Source: CAD feature listing. Evaluate the final solid. Frame: model axes, mm. A direction names the side the tool comes from. Give positions to 0.01 mm unless a question says otherwise; leave off trailing zeros. Order: outer loops, then holes, each group sorted by start corner. A loop starts at its lowest first (then second) coordinate and runs counter-clockwise, first axis right, second up. Notation, with made-up numbers: M -15,72 L 34,72 A21 ccw 34,101 Z; hole C 18,50 d8. An arc over 180 degrees is marked long. Answer in a Markdown table with one row per item. Add a question column.
(1) Section query A-A, the plane y = 31.5. Return loops of the section in (x, z).
(2) Section query C-C, the plane x = -31.5. Return loops of the section in (y, z), plus the area to 3 significant figures.
(3) Pin query (flat end, axial travel): P1, Ø2, axis at y = 27.5, z = 38.5, coming from the +X side; P2, Ø7, axis at x = -29.34, y = 31.5, coming from the -Z side; P3, Ø1, axis at y = 26.5, z = 8, coming from the -X side; P4, Ø4, axis at x = -45.74, z = 50.2, coming from the +Y side. Return the tip coordinate at first contact, or that it passes through.
(4) Mould query, pull axis Y, two halves, no side actions, for faces 1 (the face through (-47.31, 24.36, 51.75)), 2 (the face through (-28.72, 36.21, -11.17)), 3 (the face through (-29, 37.6, 11)), 4 (the face through (-31.3, 27.73, -11.33)). Classes: pulls with the +Y half, pulls with the -Y half, needs draft (parallel to the pull), parting line crosses it, or undercut.
(5) Section query B-B, the plane z = -3. Return loops of the section in (x, y), plus the area to 3 significant figures.
(6) Set-up query: faces 5 (the face through (-25, 29, -5.5)), 6 (the face through (-29, 25.1, 5)), 7 (the face through (-22.041, 31, 11)). Return all of +Z, -Z, +X, -X, +Y, -Y with unobstructed straight access to the full face (end or side cutting, diameter ignored); none if empty.
(7) Section query D-D, the plane y = 28. Return loops of the section in (x, z), plus the area to 3 significant figures.
(8) Material intervals for line 1 along Y through (x, z) = (-22, 19); line 2 along X through (y, z) = (36.75, 9.5); line 3 along Z through (x, y) = (-33, 24.5), sorted ascending.
from build123d import *

# Parameters (mm, degrees)
EXTRUDE_1_DEPTH      = 3.5
EXTRUDE_1_DEPTH_BACK = 5.5
SKETCH_1_R           = 6
SKETCH_2_R           = 4.75
EXTRUDE_2_DEPTH      = 11.5
SKETCH_3_R           = 4.25
CUT_EXTRUDE_1_DEPTH  = 11.5
SKETCH_4_W           = 14.6
SKETCH_4_H           = 12.5
EXTRUDE_3_DEPTH      = 14.2
SKETCH_5_R           = 1.25
EXTRUDE_4_DEPTH      = 1.5


with BuildPart() as part:
    # 草圖1 → 填料-伸長1 (new, two sides: drawn at the far end of the back side and taken through both)
    with BuildSketch(Plane.XY.offset(-EXTRUDE_1_DEPTH_BACK)):
        with Locations((-29.340909091, 31.5)):
            Circle(SKETCH_1_R)
    extrude(amount=EXTRUDE_1_DEPTH + EXTRUDE_1_DEPTH_BACK)

    # 草圖2 → 填料-伸長2 (add)
    with BuildSketch(Plane(origin=(0, 0, -5.5), x_dir=(-1, 0, 0), z_dir=(0, 0, -1))):
        with Locations((29.340909091, 31.5)):
            Circle(SKETCH_2_R)
    extrude(amount=EXTRUDE_2_DEPTH)

    # 草圖3 → 除料-伸長1 (cut)
    with BuildSketch(Plane(origin=(0, 0, -17), x_dir=(-1, 0, 0), z_dir=(0, 0, -1))):
        with Locations((29.340909091, 31.5)):
            Circle(SKETCH_3_R)
    extrude(amount=-CUT_EXTRUDE_1_DEPTH, mode=Mode.SUBTRACT)

    # 草圖4 → 填料-伸長3 (add)
    with BuildSketch(Plane.XY.offset(3.5)):
        with Locations((-29.340909091, 31.35)):
            Rectangle(SKETCH_4_W, SKETCH_4_H)
    extrude(amount=EXTRUDE_3_DEPTH)

    # 草圖5 → 填料-伸長4 (add)
    with BuildSketch(Plane.XZ.offset(-25.1)):
        with BuildLine():
            Line((-17.240909091, 5.697422491), (-46.240909091, 5.697422491))
            ThreePointArc((-46.240909091, 5.697422491), (-47.301569263, 6.136762319), (-47.740909091, 7.197422491))
            Line((-47.740909091, 7.197422491), (-47.740909091, 50.697422491))
            ThreePointArc((-47.740909091, 50.697422491), (-47.301569263, 51.758082663), (-46.240909091, 52.197422491))
            Line((-46.240909091, 52.197422491), (-17.240909091, 52.197422491))
            ThreePointArc((-17.240909091, 52.197422491), (-16.180248919, 51.758082663), (-15.740909091, 50.697422491))
            Line((-15.740909091, 50.697422491), (-15.740909091, 7.197422491))
            ThreePointArc((-15.740909091, 7.197422491), (-16.180248919, 6.136762319), (-17.240909091, 5.697422491))
        make_face()
        with Locations(Location((-17.740909091, 50.197422491, 0), (0, 0, 270))):
            Circle(SKETCH_5_R, mode=Mode.SUBTRACT)
        with Locations(Location((-45.740909091, 50.197422491, 0), (0, 0, 270))):
            Circle(SKETCH_5_R, mode=Mode.SUBTRACT)
    extrude(amount=EXTRUDE_4_DEPTH)


solid = part.part
Values follow:
| question | item | result |
|---|---|---|
| 1 | outline | M -36.64,3.5 L -35.34,3.5 L -35.34,-5.5 L -34.09,-5.5 L -34.09,-17 L -33.59,-17 L -33.59,-5.5 L -25.09,-5.5 L -25.09,-17 L -24.59,-17 L -24.59,-5.5 L -23.34,-5.5 L -23.34,3.5 L -22.04,3.5 L -22.04,17.7 L -36.64,17.7 Z |
| 2 | outline | M 23.6,5.7 L 25.1,5.7 L 25.1,3.5 L 25.9,3.5 L 25.9,-5.5 L 27.27,-5.5 L 27.27,-17 L 27.84,-17 L 27.84,-5.5 L 35.16,-5.5 L 35.16,-17 L 35.73,-17 L 35.73,-5.5 L 37.1,-5.5 L 37.1,3.5 L 37.6,3.5 L 37.6,17.7 L 25.1,17.7 L 25.1,52.2 L 23.6,52.2 Z |
| 2 | area | 361 mm² |
| 3 | P1 | passes through |
| 3 | P2 | stops at z = -5.5 |
| 3 | P3 | stops at x = -36.64 |
| 3 | P4 | stops at y = 25.1 |
| 4 | face 1 | needs draft |
| 4 | face 2 | parting line crosses it |
| 4 | face 3 | pulls with the +Y half |
| 4 | face 4 | undercut |
| 5 | outline | C -29.34,31.5 d12 |
| 5 | area | 113 mm² |
| 6 | face 5 | -Z |
| 6 | face 6 | -Z, +X, -X, -Y |
| 6 | face 7 | +Z, -Z, +X, +Y |
| 7 | outline | M -36.64,3.5 L -34.21,3.5 L -34.21,-5.5 L -32.55,-5.5 L -32.55,-17 L -31.75,-17 L -31.75,-5.5 L -26.93,-5.5 L -26.93,-17 L -26.13,-17 L -26.13,-5.5 L -24.47,-5.5 L -24.47,3.5 L -22.04,3.5 L -22.04,17.7 L -36.64,17.7 Z |
| 7 | area | 313 mm² |
| 8 | line 1 | y = 23.6 to 25.1 |
| 8 | line 2 | x = -36.64 to -22.04 |
| 8 | line 3 | z = 5.7 to 52.2 |
